Here's how the part is built. I have some questions about the finished solid (model axes, mm). Coordinates: 2 decimals unless noted, no trailing zeros. Loops run counter-clockwise (first coordinate to the right, second up) from the corner with the lowest first, then second, coordinate; pieces in that order, holes last. Notation, with made-up numbers: (53.5, 4) - (57.5, 4) arc R28 ccw to (57.5, 22) - close; hole circle Ø10 at (76, 54.25). An arc over 180 degrees is marked (long way). Use a Markdown table: item, result.
```python
from build123d import *

# Parameters (mm, degrees)
SKETCH_1_W      = 50
SKETCH_1_H      = 10
SKETCH_1_R      = 2.525
EXTRUDE_1_DEPTH = 4
FILLET_1_R      = 2


with BuildPart() as part:
    # 草图1 → 凸台-拉伸1 (new body)
    with BuildSketch(Plane(origin=(0, 0, 0), x_dir=(1, 0, 0), z_dir=(0, 1, 0))):
        with Locations((-20, 0)):
            Rectangle(SKETCH_1_W, SKETCH_1_H)
        Circle(SKETCH_1_R, mode=Mode.SUBTRACT)
        with Locations((-40, 0)):
            Circle(SKETCH_1_R, mode=Mode.SUBTRACT)
    extrude(amount=EXTRUDE_1_DEPTH)

    # 圆角1
    fillet_1_edges = [part.edges().sort_by_distance(p)[0] for p in [
        (-45, 2, -5),
        (5, 2, -5),
        (5, 2, 5),
        (-45, 2, 5),
    ]]
    fillet(fillet_1_edges, radius=FILLET_1_R)


solid = part.part
```
Q1. I want a section at B-B, the plane z = 0. Write out the boundary of the cut face in (x, y) (3 decimals).
Check values:
| item | result |
|---|---|
| outline | (-45, 0) - (-42.525, 0) - (-42.525, 4) - (-45, 4) - close; (-37.475, 0) - (-2.525, 0) - (-2.525, 4) - (-37.475, 4) - close; (2.525, 0) - (5, 0) - (5, 4) - (2.525, 4) - close |
Q2. I want a section at D-D, the plane z = -2. Write out the boundary of the cut face in (x, y), then the cut area to 3 significant figures.
Check values:
| item | result |
|---|---|
| outline | (-45, 0) - (-41.54, 0) - (-41.54, 4) - (-45, 4) - close; (-38.46, 0) - (-1.54, 0) - (-1.54, 4) - (-38.46, 4) - close; (1.54, 0) - (5, 0) - (5, 4) - (1.54, 4) - close |
| area | 175 mm^2 |
Q3. I want a section at C-C, the plane y = 2.2. Write out the boundary of the cut face in (x, z) (3 decimals), then the cut area to 3 significant figures.
Check values:
| item | result |
|---|---|
| outline | (-45, -3) arc R2 ccw to (-43, -5) - (3, -5) arc R2 ccw to (5, -3) - (5, 3) arc R2 ccw to (3, 5) - (-43, 5) arc R2 ccw to (-45, 3) - close; hole circle Ø5.05 at (-40, 0); hole circle Ø5.05 at (0, 0) |
| area | 457 mm^2 |
Q4. I want a section at A-A, the plane x = 0. Write out the boundary of the cut face in (y, z) (3 decimals), then the cut area to 3 significant figures.
Check values:
| item | result |
|---|---|
| outline | (0, -5) - (4, -5) - (4, -2.525) - (0, -2.525) - close; (0, 2.525) - (4, 2.525) - (4, 5) - (0, 5) - close |
| area | 19.8 mm^2 |
Q5. If we mould it in two halves opening along Z, with no side actions, what happens to faces 1 (the face through (-42.523, 1.972, -0.111)), 2 (the face through (-20, 4, 0)), 3 (the face through (-44.43, 2.03, -4.4))? For each: pulls with the +Z half, pulls with the -Z half, needs draft (parallel to the pull), parting line crosses it, or undercut.
Check values:
| item | result |
|---|---|
| face 1 | undercut |
| face 2 | needs draft |
| face 3 | pulls with the -Z half |
Q6. Please list where these lines run through material, in increasing order: L1, parallel to X at y = 0.95, z = 0 (3 decimals); L2, parallel to Z at x = -40, y = 1.65 (3 decimals); L3, parallel to X at y = 0.5, z = -1.75. Write a range as from..to.
Check values:
| item | result |
|---|---|
| L1 | -45..-42.525, -37.475..-2.525, 2.525..5 |
| L2 | -5..-2.525, 2.525..5 |
| L3 | -45..-41.82, -38.18..-1.82, 1.82..5 |
